```python
from build123d import *

# Parameters (mm, degrees)
SKETCH_1_W           = 60
SKETCH_1_H           = 60
EXTRUDE_2_DEPTH      = 30
SKETCH_3_R           = 3.5
EXTRUDE_3_DEPTH      = 7
SKETCH_4_R           = 23.5
EXTRUDE_4_DEPTH      = 2
EXTRUDE_5_DEPTH      = 7
EXTRUDE_5_DEPTH_BACK = 67
SKETCH_5_W           = 3
SKETCH_5_H           = 30


with BuildPart() as part:
    # 草图1 → 凸台-拉伸2 (new body)
    with BuildSketch(Plane(origin=(0, 0, 0), x_dir=(1, 0, 0), z_dir=(0, 1, 0))):
        Rectangle(SKETCH_1_W, SKETCH_1_H)
    extrude(amount=EXTRUDE_2_DEPTH)

    # 草图3 → 凸台-拉伸3 (add)
    with BuildSketch(Plane.XY.offset(30)):
        with Locations(Location((15, 15, 0), (0, 0, 180))):
            Circle(SKETCH_3_R)
    extrude(amount=EXTRUDE_3_DEPTH)

    # 草图4 → 凸台-拉伸4 (add)
    with BuildSketch(Plane.XY.offset(37)):
        with Locations((15, 15)):
            Circle(SKETCH_4_R)
    extrude(amount=EXTRUDE_4_DEPTH)

    # 草图5 → 凸台-拉伸5 (add, two sides: drawn at the far end of the back side and taken through both)
    with BuildSketch(Plane(origin=(30, 0, 0), x_dir=(0, 0, -1), z_dir=(1, 0, 0)).offset(-EXTRUDE_5_DEPTH_BACK)):
        with Locations((-22.5, 15)):
            Rectangle(SKETCH_5_W, SKETCH_5_H)
    extrude(amount=EXTRUDE_5_DEPTH + EXTRUDE_5_DEPTH_BACK)


solid = part.part
```
The model under review builds one solid part; all positions refer to its coordinate system, in mm. A direction names the side the tool comes from. Round coordinates to 2 decimals unless told otherwise and drop trailing zeros. Write each loop counter-clockwise with the first axis right and the second up, starting at its lowest first coordinate (ties: lowest second). Pieces come first, ordered by that corner, then holes. Notation, with made-up numbers: (53, -31) - (83, -31) arc R16 cw to (83, -15) - close; hole circle Ø9 at (-8.75, -33.5). An arc over 180 degrees is marked (long way). Answer as CSV lines item,"result". Start each with the question number.
(1) We need section B-B on x = 15. State the section outline as (y, z) points, plus the area to 3 significant figures.
(2) For pin 1 Ø5.5 at (x, y) = (33.5, 8.5) entering from -Z; pin 2 Ø10 at (x, z) = (26.5, -8.5) entering from +Y; pin 3 Ø12 at (y, z) = (31.5, -9) entering from -X, all flat-tipped, find the tip position at first contact; note any pin that passes through.
(3) For faces 1 (the flat face through (30, 15, 27)), 2 (the flat face through (-30, 15, -4)), 3 (the flat face through (-30, 15, 27)), list the 3-axis set-ups (+Z, -Z, +X, -X, +Y, -Y) from which the entire face can be reached by the end or side of a thin tool; tool diameter is ignored.
(4) We need section C-C on z = 1.5. State the section outline as (x, y) points, plus the area to 3 significant figures.
(5) To check wall thickness, follow line 1 (Z direction, x = 34, y = 26); line 2 (Z direction, x = -5, y = 10.5); line 3 (Z direction, x = 20.5, y = 36). State the ranges of each line that lie inside material, in increasing order.
(6) We need section D-D on y = 15. State the section outline as (x, z) points.
(7) Draft analysis for pull direction Z (two halves, no side actions). For faces 4 (the flat face through (0, 15, -30)), 5 (the flat face through (-1, 30, 0)), 6 (the flat face through (0, 15, 30)), state which applies: pulls with the +Z half, pulls with the -Z half, needs draft (parallel to the pull), parting line crosses it, or undercut.
(8) We need section A-A on y = 3. State the section outline as (x, z) points.
Worked answers:
1,outline,"(-8.5, 37) - (11.5, 37) - (11.5, 30) - (0, 30) - (0, -30) - (30, -30) - (30, 30) - (18.5, 30) - (18.5, 37) - (38.5, 37) - (38.5, 39) - (-8.5, 39) - close"
1,area,"1,940 mm²"
2,pin 1,"z = 21"
2,pin 2,"y = 30"
2,pin 3,"x = -30"
3,face 1,"+X, +Y, -Y"
3,face 2,"-Z, -X, +Y, -Y"
3,face 3,"+Z, -X, +Y, -Y"
4,outline,"(-30, 0) - (30, 0) - (30, 30) - (-30, 30) - close"
4,area,"1,800 mm²"
5,line 1,"21 to 24, 37 to 39"
5,line 2,"-30 to 30, 37 to 39"
5,line 3,"37 to 39"
6,outline,"(-37, 21) - (-30, 21) - (-30, -30) - (30, -30) - (30, 21) - (37, 21) - (37, 24) - (30, 24) - (30, 30) - (18.5, 30) - (18.5, 37) - (38.5, 37) - (38.5, 39) - (-8.5, 39) - (-8.5, 37) - (11.5, 37) - (11.5, 30) - (-30, 30) - (-30, 24) - (-37, 24) - close"
7,face 4,"pulls with the -Z half"
7,face 5,"needs draft"
7,face 6,"undercut"
8,outline,"(-37, 21) - (-30, 21) - (-30, -30) - (30, -30) - (30, 21) - (37, 21) - (37, 24) - (30, 24) - (30, 30) - (-30, 30) - (-30, 24) - (-37, 24) - close; (-5.21, 37) - (35.21, 37) - (35.21, 39) - (-5.21, 39) - close"
